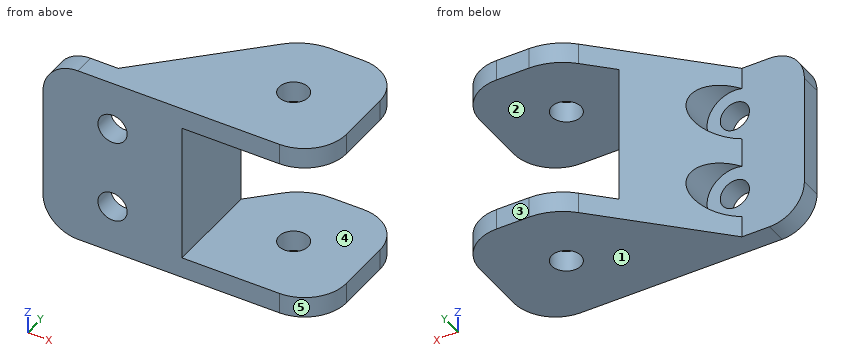
```python
from build123d import *

# Parameters (mm, degrees)
SKETCH_1_R          = 2.1
EXTRUDE_1_DEPTH     = 3
SKETCH_3_W          = 20
SKETCH_3_H          = 3
EXTRUDE_2_DEPTH     = 20
FILLET_2_R          = 6
CHAMFER_2_SIZE      = 6
FILLET_3_R          = 8
EXTRUDE_5_DEPTH     = 26
SKETCH_12_R         = 2.1
CUT_EXTRUDE_4_DEPTH = 30
SKETCH_13_R         = 4
CUT_EXTRUDE_5_DEPTH = 30


with BuildPart() as part:
    # 草图1 → 凸台-拉伸1 (new body)
    with BuildSketch(Plane(origin=(0, 0, 0), x_dir=(1, 0, 0), z_dir=(0, 1, 0))):
        with BuildLine():
            Line((0, 0), (-15, 0))
            ThreePointArc((-15, 0), (-18.535533906, 1.464466094), (-20, 5))
            Line((-20, 5), (-20, 21))
            ThreePointArc((-20, 21), (-18.535533906, 24.535533906), (-15, 26))
            Line((-15, 26), (0, 26))
            Line((0, 26), (0, 0))
        make_face()
        with Locations(Location((-10, 19, 0), (0, 0, 270))):
            Circle(SKETCH_1_R, mode=Mode.SUBTRACT)
        with Locations(Location((-10, 7, 0), (0, 0, 270))):
            Circle(SKETCH_1_R, mode=Mode.SUBTRACT)
    extrude(amount=EXTRUDE_1_DEPTH)

    # 草图3 → 凸台-拉伸2 (add)
    with BuildSketch(Plane(origin=(0, 0, 0), x_dir=(1, 0, 0), z_dir=(0, 1, 0))):
        with Locations((10, 24.5)):
            Rectangle(SKETCH_3_W, SKETCH_3_H)
        with Locations((10, 1.5)):
            Rectangle(SKETCH_3_W, SKETCH_3_H)
    extrude(amount=EXTRUDE_2_DEPTH)

    # 圆角2
    fillet_2_edges = [part.edges().sort_by_distance(p)[0] for p in [
        (20, 0, -24.5),
        (20, 20, -24.5),
        (20, 0, -1.5),
        (20, 20, -1.5),
    ]]
    fillet(fillet_2_edges, radius=FILLET_2_R)

    # 倒角2
    chamfer_2_edges = [part.edges().sort_by_distance(p)[0] for p in [
        (0, 20, -24.5),
        (0, 20, -1.5),
    ]]
    chamfer(chamfer_2_edges, length=CHAMFER_2_SIZE)

    # 圆角3
    fillet_3_edges = [part.edges().sort_by_distance(p)[0] for p in [
        (6, 20, -1.5),
        (6, 20, -24.5),
    ]]
    fillet(fillet_3_edges, radius=FILLET_3_R)

    # 草图8 → 凸台-拉伸5 (add)
    with BuildSketch(Plane(origin=(0, 0, -26), x_dir=(-1, 0, 0), z_dir=(0, 0, -1))):
        Polygon((0, 14), (11, 3), (0, 3), align=None)
    extrude(amount=-EXTRUDE_5_DEPTH)

    # 草图12 → 切除-拉伸4 (cut)
    with BuildSketch(Plane.XY):
        with Locations((10, 10)):
            Circle(SKETCH_12_R)
    extrude(amount=-CUT_EXTRUDE_4_DEPTH, mode=Mode.SUBTRACT)

    # 草图13 → 切除-拉伸5 (cut)
    with BuildSketch(Plane(origin=(0, 3, 0), x_dir=(1, 0, 0), z_dir=(0, 1, 0))):
        with Locations((-10, 19)):
            Circle(SKETCH_13_R)
        with Locations((-10, 7)):
            Circle(SKETCH_13_R)
    extrude(amount=CUT_EXTRUDE_5_DEPTH, mode=Mode.SUBTRACT)


solid = part.part
```
CAD build for the part. Positions are in the model's coordinates, mm. Face numbers are marked on the shaded views. A direction names the side the tool comes from. Coordinates: 2 decimals unless noted, no trailing zeros. Loops run counter-clockwise (first coordinate to the right, second up) from the corner with the lowest first, then second, coordinate; pieces in that order, holes last. Notation, with made-up numbers: (56, -16) - (79, -16) arc R32 cw to (79, 13) - close; hole circle Ø4 at (-10.5, -25). An arc over 180 degrees is marked (long way). Return JSON: item names as keys, results as strings.
1. Probe L1, parallel to Z at x = 11, y = 8; L2, parallel to Y at x = 10, z = -2.35; L3, parallel to Y at x = -18, z = -23.75. List the from-to ranges inside material, lowest first. Write a range as from..to.
Result:
{"L1": "z = -26..-23, -3..0", "L2": "y = 0..7.9, 12.1..20", "L3": "y = 0..3"}
2. Band-saw the part on D-D (x = 4.5). Give the cut face in (y, z), and give its area (3 significant figures).
Result:
{"outline": "(0, -26) - (18.39, -26) - (18.39, -23) - (0, -23) - close; (0, -3) - (18.39, -3) - (18.39, 0) - (0, 0) - close", "area": "110 mm2"}
3. Band-saw the part on C-C (z = -19). Give the cut face in (x, y).
Result:
{"outline": "(-20, 0) - (-12.1, 0) - (-12.1, 3) - (-20, 3) - close; (-7.9, 0) - (0, 0) - (0, 14) - (-6, 8) - (-6, 3) - (-7.9, 3) - close"}
4. 3-axis set-ups, long thin cutter, end or side, ignore diameter. For the marked faces 4 and 5: which of +Z, -Z, +X, -X, +Y, -Y reach the whole face in a straight line?
Result:
{"face 4": "+X, +Y, -Y", "face 5": "+Z, -Z, +X, -Y"}
5. Band-saw the part on B-B (y = 10). Give the cut face in (x, z).
Result:
{"outline": "(-4, -26) - (7.9, -26) - (7.9, -23) - (0, -23) - (0, -3) - (7.9, -3) - (7.9, 0) - (-4, 0) - close; (12.1, -26) - (20, -26) - (20, -23) - (12.1, -23) - close; (12.1, -3) - (20, -3) - (20, 0) - (12.1, 0) - close"}
6. Band-saw the part on A-A (x = 10). Give the cut face in (y, z).
Result:
{"outline": "(0, -26) - (7.9, -26) - (7.9, -23) - (0, -23) - close; (0, -3) - (7.9, -3) - (7.9, 0) - (0, 0) - close; (12.1, -26) - (20, -26) - (20, -23) - (12.1, -23) - close; (12.1, -3) - (20, -3) - (20, 0) - (12.1, 0) - close"}
7. Mould opens along Z. For the marked faces 1, 2 and 3 say: released by +Z, released by -Z, zero draft, split by the parting line, or undercut.
Result:
{"face 1": "released by -Z", "face 2": "undercut", "face 3": "zero draft"}
8. Drop flat-ended pins along their axis: pin 1 (15.5 mm diameter, centred on x = -15, z = -13.5, fed in from +Y); pin 2 (5 mm diameter, centred on x = -10, z = -7, fed in from +Y); pin 3 (1 mm diameter, centred on y = 2, z = -3, fed in from +X). Give the stop position or say it passes through.
Result:
{"pin 1": "stops at y = 6.75", "pin 2": "stops at y = 3", "pin 3": "stops at x = 18.87"}
